from build123d import *

# Parameters (mm, degrees)
F0_W     = 50.5
F0_H     = 50.5
F1_DEPTH = 2
F2_W     = 45.2
F2_H     = 45.2
F3_DEPTH = 5
F4_W     = 42
F4_H     = 42
F5_DEPTH = 5
F6_R     = 2.5
F7_R     = 2
F8_SIZE  = 1
F9_R     = 1


with BuildPart() as f1:
    # F0 (on Top) → F1 (new body)
    with BuildSketch(Plane.XY):
        Rectangle(F0_W, F0_H)
    extrude(amount=F1_DEPTH)

    # F2 (on face) → F3 (join)
    with BuildSketch(Plane.XY.offset(2)):
        Rectangle(F2_W, F2_H)
    extrude(amount=F3_DEPTH)

    # F4 (on face) → F5 (cut, through all)
    with BuildSketch(Plane.XY.offset(2)):
        Rectangle(F4_W, F4_H)
    extrude(amount=F5_DEPTH, mode=Mode.SUBTRACT)

    # F6
    f6_edges = [f1.edges().sort_by_distance(p)[0] for p in [
        (-25.25, 25.25, 1),
        (-25.25, -25.25, 1),
        (25.25, -25.25, 1),
        (25.25, 25.25, 1),
        (-22.6, 22.6, 4.5),
        (-22.6, -22.6, 4.5),
        (22.6, -22.6, 4.5),
        (22.6, 22.6, 4.5),
    ]]
    fillet(f6_edges, radius=F6_R)

    # F7
    f7_edges = [f1.edges().sort_by_distance(p)[0] for p in [
        (-21, 21, 4.5),
        (21, 21, 4.5),
        (21, -21, 4.5),
        (-21, -21, 4.5),
    ]]
    fillet(f7_edges, radius=F7_R)

    # F8
    f8_edges = [f1.edges().sort_by_distance(p)[0] for p in [
        (-22.6, 0, 7),
    ]]
    chamfer(f8_edges, length=F8_SIZE)

    # F9
    f9_edges = [f1.edges().sort_by_distance(p)[0] for p in [
        (0, 25.25, 0),
    ]]
    fillet(f9_edges, radius=F9_R)


solid = f1.part
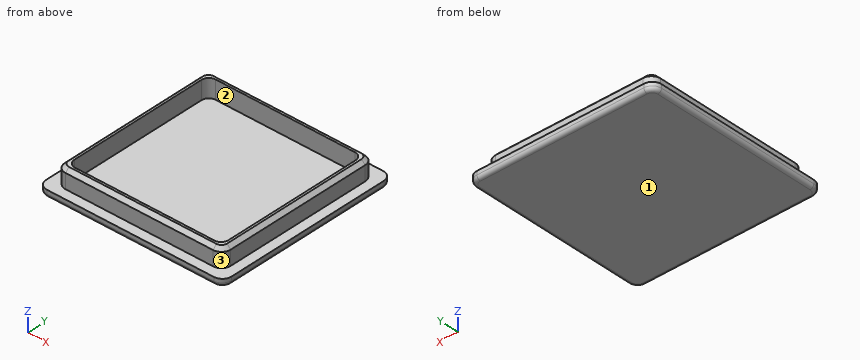
Can you work these out from the model? Positions are in its coordinate system, mm. Face numbers are marked on the shaded views. Round coordinates to 2 decimals unless told otherwise and drop trailing zeros. Write each loop counter-clockwise with the first axis right and the second up, starting at its lowest first coordinate (ties: lowest second). Pieces come first, ordered by that corner, then holes. Notation, with made-up numbers: (19, -17) -> (47, -17) arc R18 ccw to (47, -1) -> close; hole circle Ø9 at (-14.5, -18.5). An arc over 180 degrees is marked (long way). One line per question, with ' | ' between items. Start each with the question number.
1) Suppose I cut it at A-A on z = 4.25. Write out the boundary of the cut face in (x, y).
2) I'm going to push flat-ended pins straight in: P1, Ø12, axis at x = 2, y = -10.5, coming from the +Z side; P2, Ø2.5, axis at x = 2, z = 4, coming from the +Y side; P3, Ø3, axis at x = -0.5, z = 3, coming from the +Y side; P4, Ø2, axis at y = -9, z = 3.5, coming from the -X side. Where does each tip first touch, or does it pass through?
3) Suppose I cut it at B-B on x = -0.5. Write out the boundary of the cut face in (y, z).
4) I need wall thicknesses on line 1 (X direction, y = -16, z = 2.75); line 2 (Z direction, x = -12.5, y = 14). Which ranges of each line are inside material? Lowest first, please. Write a range as [from, to].
5) If we mould it in two halves opening along Y, with no side actions, what happens to the marked faces 1, 2 and 3? For each: released by +Y, released by -Y, zero draft, split by the parting line, or undercut.
Return value:
1) outline: (-22.6, -20.1) arc R2.5 ccw to (-20.1, -22.6) -> (20.1, -22.6) arc R2.5 ccw to (22.6, -20.1) -> (22.6, 20.1) arc R2.5 ccw to (20.1, 22.6) -> (-20.1, 22.6) arc R2.5 ccw to (-22.6, 20.1) -> close; hole (-21, -19) arc R2 ccw to (-19, -21) -> (19, -21) arc R2 ccw to (21, -19) -> (21, 19) arc R2 ccw to (19, 21) -> (-19, 21) arc R2 ccw to (-21, 19) -> close
2) P1: stops at z = 2 | P2: stops at y = 22.6 | P3: stops at y = 25.25 | P4: stops at x = -22.6
3) outline: (-25.25, 1) arc R1 ccw to (-24.25, 0) -> (24.25, 0) arc R1 ccw to (25.25, 1) -> (25.25, 2) -> (22.6, 2) -> (22.6, 6) -> (21.6, 7) -> (21, 7) -> (21, 2) -> (-21, 2) -> (-21, 7) -> (-21.6, 7) -> (-22.6, 6) -> (-22.6, 2) -> (-25.25, 2) -> close
4) line 1: x = [-22.6, -21], [21, 22.6] | line 2: z = [0, 2]
5) face 1: zero draft | face 2: undercut | face 3: released by -Y
